For this review, use the dimensioned drawing (mm, ordinates from the lowest corner) and the shaded views. Coordinates: 2 decimals unless noted, no trailing zeros. Loops run counter-clockwise (first coordinate to the right, second up) from the corner with the lowest first, then second, coordinate; pieces in that order, holes last. Notation, with made-up numbers: M 87.25,-23.5 L 117.25,-23.5 A32 ccw 117.25,9.5 Z; hole C 39.5,0 d9. An arc over 180 degrees is marked long. Write item = value, one per line. Start each with the question number.
Q1. Clearance check with flat-ended pins moving along their axes: pin 1 Ø1.5 at (y, z) = (151.5, 2) entering from -X; pin 2 Ø0.8 at (x, z) = (7, 2.5) entering from -Y; pin 3 Ø1.9 at (y, z) = (140, 4) entering from +X. State where each tip first meets the part, or that it passes through.
Q2. We need section B-B on y = 106. Give the boundary of the cut face in (x, z), and give its area (3 significant figures).
Q3. We need section A-A on z = 4. Give the boundary of the cut face in (x, y).
Q4. We need section D-D on y = 16. Give the boundary of the cut face in (x, z), and give its area (3 significant figures).
Q5. Wall thickness on probe 1 along Y at (x, z) = (7, 3.5); probe 2 along X at (y, z) = (109, 4.5); probe 3 along X at (y, z) = (68.5, 6.5): over which ranges is each line inside the solid? List them lowest first.
Q6. We need section C-C on x = 2.75. Give the boundary of the cut face in (y, z), and give its area (3 significant figures).
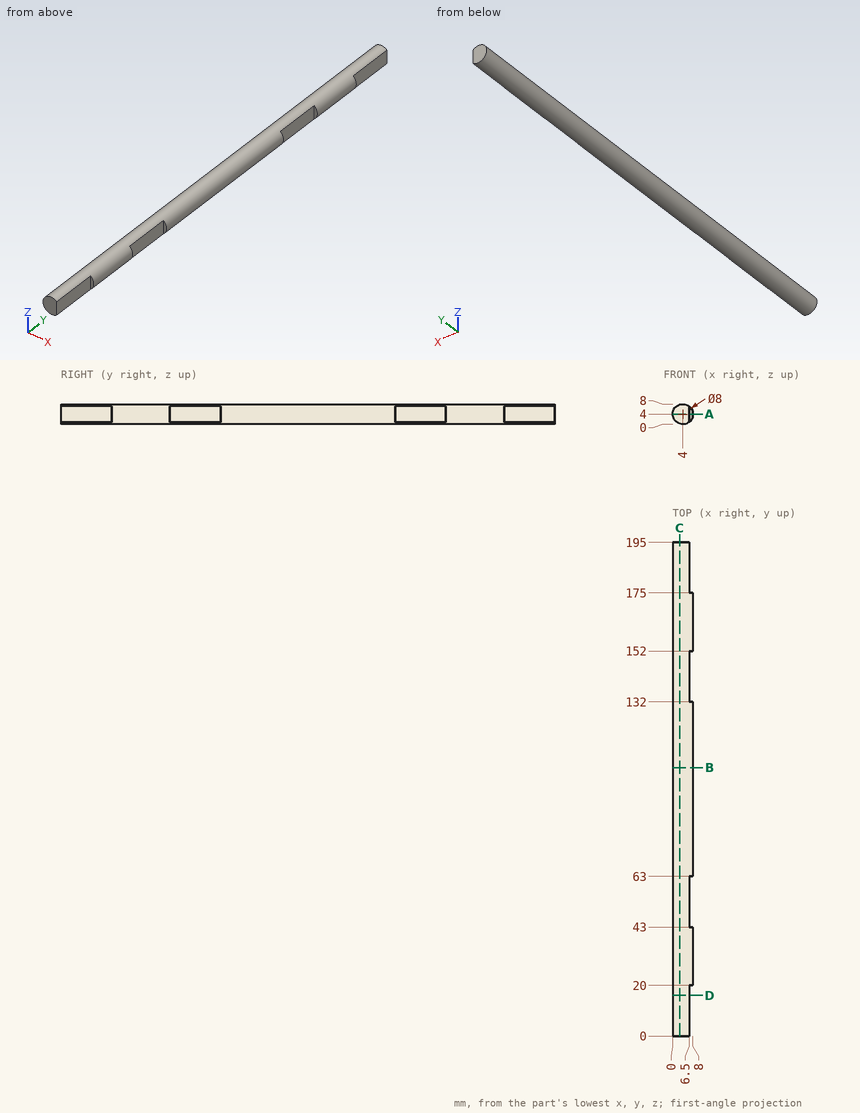
Returned:
q1.pin_1 = 0.2
q1.pin_2 = 20
q1.pin_3 = 6.5
q2.outline = C 4,4 d8
q2.area = 50.3 mm^2
q3.outline = M 0,0 L 6.5,0 L 6.5,20 L 8,20 L 8,43 L 6.5,43 L 6.5,63 L 8,63 L 8,132 L 6.5,132 L 6.5,152 L 8,152 L 8,175 L 6.5,175 L 6.5,195 L 0,195 Z
q4.outline = M 6.5,0.88 L 6.5,7.12 A4 ccw long Z
q4.area = 43.7 mm^2
q5.probe_1 = 20 to 43, 63 to 132, 152 to 175
q5.probe_2 = 0.03 to 7.97
q5.probe_3 = 0.88 to 7.12
q6.outline = M 0,0.2 L 195,0.2 L 195,7.8 L 0,7.8 Z
q6.area = 1,480 mm^2
